Autodesk Inventor part; units mm, degrees
ref_plane "РабПлоскость1" through (0, 0, 0) normal (0, 0, 1) x (1, 0, 0)
ref_plane "YZ Plane" through (0, 0, 0) normal (1, 0, 0) x (0, 1, 0)
ref_plane "XZ Plane" through (0, 0, 0) normal (0, 1, 0) x (-1, 0, 0)
sketch "Эскиз1" plane through (0, 0, 0) normal (0, 0, 1) x (1, 0, 0)
  line L0 (-5, 5) -> (5, 5)
  line L1 (5, 5) -> (5, -5)
  line L2 (5, -5) -> (-5, -5)
  line L3 (-5, -5) -> (-5, 5)
  point P0 (0, 0)
  point P1 (0, 5)
  point P2 (5, 0)
  dimension "d0" = 10
  dimension "d1" = 10
extrude "Выдавливание1" add sketch "Эскиз1" against normal blind 10
sketch "Эскиз2" plane through (0, 0, 0) normal (0, 0, 1) x (1, 0, 0)
  line L0 (-4.6144, 4.1403) -> (8.1453, 4.1403) construction
  line L1 (8.1453, 4.1403) -> (8.1453, 2.1383) construction
  line L2 (8.1453, 2.1383) -> (-4.6144, 2.1383) construction
  line L3 (-4.6144, 2.1383) -> (-4.6144, 4.1403) construction
  point P0 (0, 0)
ref_plane "РабПлоскость1" through (0, 0, 0) normal (0, 0, 1) x (1, 0, 0)
sketch "Эскиз3" plane through (0, 0, 0) normal (0, 0, 1) x (1, 0, 0)
  circle A0 centre (-2.2997, -3.0689) radius 0.5
  circle A1 centre (3.0277, -3.0689) radius 0.5
  point P0 (0, 0)
  dimension "d5" = 1
  dimension "d6" = 1
extrude "Выдавливание2" add sketch "Эскиз3" along normal blind 0.3
sketch "Эскиз4" plane through (0, 0, 0) normal (0, 0, 1) x (1, 0, 0)
  circle A0 centre (-2.2997, -3.0689) radius 0.5
  circle A1 centre (-2.2997, -3.0689) radius 0.1
  circle A2 centre (3.039, -3.0689) radius 0.1
  point P0 (0, 0)
  dimension "d9" = 0.2
  dimension "d10" = 0.2
extrude "Выдавливание3" add sketch "Эскиз4" along normal blind 0.4 contours A1 | A2
properties part number "rf-generator"
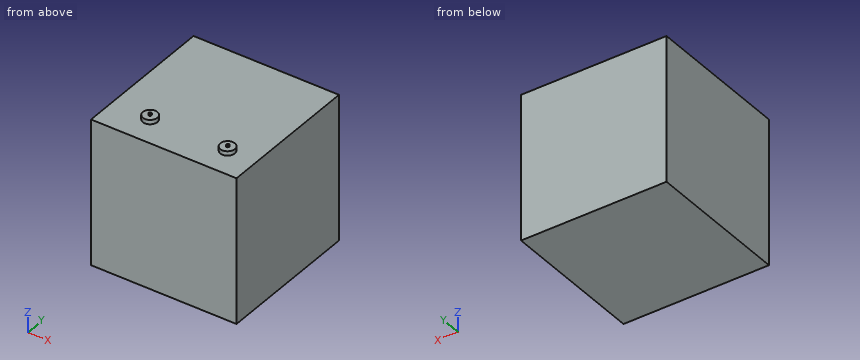
Check sheet for the modelled part. Datum: model origin and axes. Units: mm. Round coordinates to 2 decimals unless told otherwise and drop trailing zeros. Loops run counter-clockwise (first coordinate to the right, second up) from the corner with the lowest first, then second, coordinate; pieces in that order, holes last. Notation, with made-up numbers: M -18.75,18.5 L 36.25,18.5 A23 cw 36.25,39.5 Z; hole C -34,-4.5 d3. An arc over 180 degrees is marked long. One line per item, written item: value.
(1) Thickness scan on line 1 (Z direction, x = 0.5, y = 3.25). Record the ranges inside material, lowest first.
Computed values:
line 1: z = -10 to 0
(2) Sectioned sample at A-A, the plane x = -0.25. Record the cut outline in (y, z).
Computed values:
outline: M -5,-10 L 5,-10 L 5,0 L -5,0 Z
(3) Depth check by flat-ended pin: pin 1 Ø2 at (x, y) = (1.5, 2) entering from +Z. Enter the tip coordinate at first touch or a pass-through.
Computed values:
pin 1: stops at z = 0
